Source: CAD feature listing. Evaluate the final solid. Frame: model axes, mm. Face numbers are marked on the shaded views. A direction names the side the tool comes from. Round coordinates to 2 decimals unless told otherwise and drop trailing zeros. Order: outer loops, then holes, each group sorted by start corner. A loop starts at its lowest first (then second) coordinate and runs counter-clockwise, first axis right, second up. Notation, with made-up numbers: (12, 7) -> (69, 7) arc R23 cw to (69, 43) -> close; hole circle Ø1 at (53, -17.75). An arc over 180 degrees is marked (long way). Use a Markdown table: item, result. Add a question column.
```python
from build123d import *

# Parameters (mm, degrees)
F1_DEPTH       = 304.8
F4_D           = 10.0838
F4_DEPTH       = 20.6502
F4_TIP         = 3.0294791551
F4_ON_F2_D     = 10.0838
F4_ON_F2_DEPTH = 20.6502
F4_ON_F2_TIP   = 3.0294791551


with BuildPart() as f1:
    # F0 (on Front) → F1 (new body)
    with BuildSketch(Plane.XZ):
        Polygon((0, 50.8), (0, 0), (50.8, 0), (50.8, 6.35), (6.35, 6.35), (6.35, 50.8), align=None)
    extrude(amount=F1_DEPTH)

    # F4
    with Locations(Plane.XY.offset(6.35)):
        with Locations((28.575, -152.4), (28.575, -25.4), (28.575, -279.4)):
            Hole(F4_D / 2, depth=F4_DEPTH)
            with Locations((0, 0, -(F4_DEPTH + F4_TIP / 2))):  # 118° drill point
                Cone(0, F4_D / 2, F4_TIP, mode=Mode.SUBTRACT)

    # F4 on F2
    with Locations(Plane.YZ.offset(6.35)):
        with Locations((-279.4, 28.575), (-152.4, 28.575), (-25.4, 28.575)):
            Hole(F4_ON_F2_D / 2, depth=F4_ON_F2_DEPTH)
            with Locations((0, 0, -(F4_ON_F2_DEPTH + F4_ON_F2_TIP / 2))):  # 118° drill point
                Cone(0, F4_ON_F2_D / 2, F4_ON_F2_TIP, mode=Mode.SUBTRACT)


solid = f1.part
```
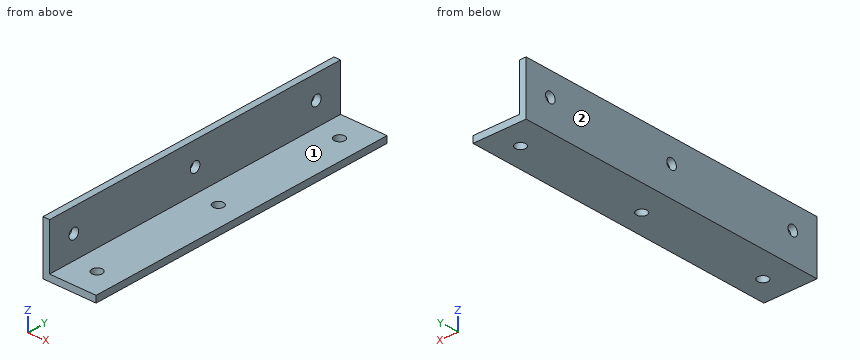
1) Line query: probe 1 along Z at (x, y) = (13.5, -102.5); probe 2 along X at (y, z) = (-279, 3). Output: solid intervals per line, ascending. Write a range as from..to.
2) Section B-B on x = 30. Output: boundary loops of the cut face in (y, z).
3) Section C-C on z = 17.5. Output: boundary loops of the cut face in (x, y).
4) Section A-A on y = -152.4. Output: boundary loops of the cut face in (x, z).
5) Reachability of the marked faces 1 and 2 from +Z, -Z, +X, -X, +Y, -Y: full face, straight path, thin tool, end or side. Return the list, or none.
6) First-contact query: pin 1 Ø16 at (x, y) = (28.575, -25.4) entering from +Z; pin 2 Ø10 at (y, z) = (-219, 43.5) entering from +X. Flat tips, straight axial feed; report the tip coordinate or a pass-through.
7) Section D-D on y = -76.5. Output: boundary loops of the cut face in (x, z).
Conclusion:
| question | item | result |
|---|---|---|
| 1 | probe 1 | z = 0..6.35 |
| 1 | probe 2 | x = 0..23.55, 33.6..50.8 |
| 2 | outline | (-304.8, 0) -> (-284.24, 0) -> (-284.24, 6.35) -> (-304.8, 6.35) -> close; (-274.56, 0) -> (-157.24, 0) -> (-157.24, 6.35) -> (-274.56, 6.35) -> close; (-147.56, 0) -> (-30.24, 0) -> (-30.24, 6.35) -> (-147.56, 6.35) -> close; (-20.56, 0) -> (0, 0) -> (0, 6.35) -> (-20.56, 6.35) -> close |
| 3 | outline | (0, -304.8) -> (6.35, -304.8) -> (6.35, 0) -> (0, 0) -> close |
| 4 | outline | (0, 0) -> (23.53, 0) -> (23.53, 6.35) -> (6.35, 6.35) -> (6.35, 23.53) -> (0, 23.53) -> close; (0, 33.62) -> (6.35, 33.62) -> (6.35, 50.8) -> (0, 50.8) -> close; (33.62, 0) -> (50.8, 0) -> (50.8, 6.35) -> (33.62, 6.35) -> close |
| 5 | face 1 | +Z, +X, +Y, -Y |
| 5 | face 2 | +Z, -Z, -X, +Y, -Y |
| 6 | pin 1 | stops at z = 6.35 |
| 6 | pin 2 | stops at x = 6.35 |
| 7 | outline | (0, 0) -> (50.8, 0) -> (50.8, 6.35) -> (6.35, 6.35) -> (6.35, 50.8) -> (0, 50.8) -> close |
